The model under review builds one solid part; all positions refer to its coordinate system, in mm. A direction names the side the tool comes from. Round coordinates to 2 decimals unless told otherwise and drop trailing zeros. Loops run counter-clockwise (first coordinate to the right, second up) from the corner with the lowest first, then second, coordinate; pieces in that order, holes last. Notation, with made-up numbers: (-22.5, 47.5) -> (21.5, 47.5) arc R17 ccw to (21.5, 59.5) -> close; hole circle Ø7 at (-16.5, 79). An arc over 180 degrees is marked (long way). Use a Markdown table: item, result. Add a question column.
1) For faces 1 (the cylindrical face through (-0.325, 15.964, 0.493)), 2 (the flat face through (0, 9, 0)), list the 3-axis set-ups (+Z, -Z, +X, -X, +Y, -Y) from which the entire face can be reached by the end or side of a thin tool; tool diameter is ignored.
2) Consider section B-B on y = 14.5. Give the boundary of the cut face in (x, z).
3) Mouldability with a two-part tool opening along X and no side actions: class faces 3 (the cylindrical face through (1.5, 3.57, 0.49)), 4 (the flat face through (-5, 9, -3)), 5 (the flat face through (4, 8.9, 0.5)), 6 (the cylindrical face through (-4.49, 13, -3.93)) as released by +X, released by -X, zero draft, split by the parting line, or undercut.
4) Insertion check: pin 1 (2.5 mm diameter, centred on x = 1.5, y = 9, fed in from -Z); pin 2 (1.5 mm diameter, centred on x = -0.5, y = 14, fed in from +Z); pin 3 (4 mm diameter, centred on y = 14.5, z = -4, fed in from +X). Each pin has a flat end and moves straight along its axis. Give the tip position at first contact, or say it passes through.
5) Consider section A-A on x = 0. Give the boundary of the cut face in (y, z), plus the area to 3 significant figures.
6) Consider section D-D on y = 7.25. Give the boundary of the cut face in (x, z), plus the area to 3 significant figures.
7) Consider section C-C on z = -5.25. Give the boundary of the cut face in (x, y), plus the area to 3 significant figures.
8) Wall thickness on probe 1 along Y at (x, z) = (0, 0.65); probe 2 along Z at (x, y) = (-4.6, 3.5); probe 3 along X at (y, z) = (14.5, 0.6): over which ranges is each line inside the solid? List them lowest first.
from build123d import *

# Parameters (mm, degrees)
ESQUISSE1_W             = 8
ESQUISSE1_H             = 18
BOSS_EXTRU_1_DEPTH      = 1
ESQUISSE2_W             = 1
ESQUISSE2_H             = 18
BOSS_EXTRU_2_DEPTH      = 9
ESQUISSE3_R             = 1.5
ENL_V_MAT_EXTRU_1_DEPTH = 22.260291625
ESQUISSE4_R             = 1.5
ENL_V_MAT_EXTRU_2_DEPTH = 21.322401433


with BuildPart() as part:
    # Esquisse1 → Boss.-Extru.1 (new body)
    with BuildSketch(Plane.XY):
        with Locations((0, 9)):
            Rectangle(ESQUISSE1_W, ESQUISSE1_H)
    extrude(amount=BOSS_EXTRU_1_DEPTH)

    # Esquisse2 → Boss.-Extru.2 (add)
    with BuildSketch(Plane.XY.offset(1)):
        with Locations((-4.5, 9)):
            Rectangle(ESQUISSE2_W, ESQUISSE2_H)
    extrude(amount=-BOSS_EXTRU_2_DEPTH)

    # Esquisse3 → Enlèv. mat.-Extru.1 (cut, through all)
    with BuildSketch(Plane(origin=(-4, 0, 0), x_dir=(0, 0, -1), z_dir=(1, 0, 0))):
        with Locations(Location((4, 14.5, 0), (0, 0, 90))):
            Circle(ESQUISSE3_R)
        with Locations(Location((4, 3.5, 0), (0, 0, 270))):
            Circle(ESQUISSE3_R)
    extrude(amount=-ENL_V_MAT_EXTRU_1_DEPTH, mode=Mode.SUBTRACT)

    # Esquisse4 → Enlèv. mat.-Extru.2 (cut, through all)
    with BuildSketch(Plane(origin=(0, 0, 0), x_dir=(-1, 0, 0), z_dir=(0, 0, -1))):
        with Locations((0, 3.5)):
            Circle(ESQUISSE4_R)
        with Locations(Location((0, 14.5, 0), (0, 0, 180))):
            Circle(ESQUISSE4_R)
    extrude(amount=-ENL_V_MAT_EXTRU_2_DEPTH, mode=Mode.SUBTRACT)


solid = part.part
Result set:
| question | item | result |
|---|---|---|
| 1 | face 1 | +Z, -Z |
| 1 | face 2 | -Z, +X, +Y, -Y |
| 2 | outline | (-5, -8) -> (-4, -8) -> (-4, -5.5) -> (-5, -5.5) -> close; (-5, -2.5) -> (-4, -2.5) -> (-4, 0) -> (-1.5, 0) -> (-1.5, 1) -> (-5, 1) -> close; (1.5, 0) -> (4, 0) -> (4, 1) -> (1.5, 1) -> close |
| 3 | face 3 | undercut |
| 3 | face 4 | released by -X |
| 3 | face 5 | released by +X |
| 3 | face 6 | zero draft |
| 4 | pin 1 | z = 0 |
| 4 | pin 2 | through |
| 4 | pin 3 | x = -4 |
| 5 | outline | (0, 0) -> (2, 0) -> (2, 1) -> (0, 1) -> close; (5, 0) -> (13, 0) -> (13, 1) -> (5, 1) -> close; (16, 0) -> (18, 0) -> (18, 1) -> (16, 1) -> close |
| 5 | area | 12.0 mm2 |
| 6 | outline | (-5, -8) -> (-4, -8) -> (-4, 0) -> (4, 0) -> (4, 1) -> (-5, 1) -> close |
| 6 | area | 17.0 mm2 |
| 7 | outline | (-5, 0) -> (-4, 0) -> (-4, 2.67) -> (-5, 2.67) -> close; (-5, 4.33) -> (-4, 4.33) -> (-4, 13.67) -> (-5, 13.67) -> close; (-5, 15.33) -> (-4, 15.33) -> (-4, 18) -> (-5, 18) -> close |
| 7 | area | 14.7 mm2 |
| 8 | probe 1 | 0 to 2, 5 to 13, 16 to 18 |
| 8 | probe 2 | -8 to -5.5, -2.5 to 1 |
| 8 | probe 3 | -5 to -1.5, 1.5 to 4 |
